Geometry check sheet. Reference: the model listing, model coordinates, mm. A direction names the side the tool comes from. Round coordinates to 2 decimals unless told otherwise and drop trailing zeros. Write each loop counter-clockwise with the first axis right and the second up, starting at its lowest first coordinate (ties: lowest second). Pieces come first, ordered by that corner, then holes. Notation, with made-up numbers: M 18.25,36.5 L 26.25,36.5 A21 ccw 26.25,44.5 Z; hole C -30,51 d8. An arc over 180 degrees is marked long. Use a Markdown table: item, result.
```python
from build123d import *

# Parameters (mm, degrees)
SKETCH1_R           = 6.477
SKETCH1_R_2         = 3.175
BOSS_EXTRUDE1_DEPTH = 228.6
SKETCH2_W           = 12.954
SKETCH2_H           = 7.9375
CUT_EXTRUDE1_DEPTH  = 229.783441398


with BuildPart() as part:
    # Sketch1 → Boss-Extrude1 (new body)
    with BuildSketch(Plane.XY):
        Circle(SKETCH1_R)
        Circle(SKETCH1_R_2, mode=Mode.SUBTRACT)
    extrude(amount=BOSS_EXTRUDE1_DEPTH)

    # Sketch2 → Cut-Extrude1 (cut, through all)
    with BuildSketch(Plane(origin=(0, 0, 0), x_dir=(1, 0, 0), z_dir=(0, 1, 0))):
        with Locations((0, -188.11875)):
            Rectangle(SKETCH2_W, SKETCH2_H)
    extrude(amount=-CUT_EXTRUDE1_DEPTH, mode=Mode.SUBTRACT)


solid = part.part
```
Item 1: Cross-section at B-B, the plane z = 174. Record the cut outline in (x, y) (3 decimals).
Outcome:
| item | result |
|---|---|
| outline | C 0,0 d12.954; hole C 0,0 d6.35 |
Item 2: Access from +Z, -Z, +X, -X, +Y, -Y to the whole of each face (thin tool, end or side, straight path). Record for faces 5 (the face through (-0.843, 6.422, 112.7)), 6 (the face through (0, -4, 184.15)).
Outcome:
| item | result |
|---|---|
| face 5 | +Z, -Z |
| face 6 | +X, -X, -Y |
Item 3: Mould release check, pull along Z, two halves, no side actions. Record for faces 1 (the face through (-0.41, 3.15, 112.7)), 2 (the face through (0, -4, 192.088)), 3 (the face through (3, 2, 0)), 4 (the face through (3, 2, 228.6)): +Z half, -Z half, draft (parallel to the pull), parting line (faces both ways), or undercut.
Outcome:
| item | result |
|---|---|
| face 1 | draft |
| face 2 | undercut |
| face 3 | -Z half |
| face 4 | +Z half |
Item 4: Material ranges on line 1 along Z through (x, y) = (-4.5, -3); line 2 along Y through (x, z) = (0, 170) (3 decimals), recorded low to high. Write a range as from..to.
Outcome:
| item | result |
|---|---|
| line 1 | z = 0..184.15, 192.09..228.6 |
| line 2 | y = -6.477..-3.175, 3.175..6.477 |
Item 5: Cross-section at A-A, the plane x = 0. Count the separate pieces of the cut face and the enclosed holes in it, and give its area (3 significant figures).
Outcome:
| item | result |
|---|---|
| separate pieces | 3 |
| enclosed holes | 0 |
| area | 1,480 mm2 |
Item 6: Go/stop test with flat-tipped pins: pin 1 (2 mm diameter, centred on y = -3, z = 43.5, fed in from +X); pin 2 (3.5 mm diameter, centred on x = 4.5, z = 186.5, fed in from -Y); pin 3 (1 mm diameter, centred on x = -1, z = 204, fed in from +Y). Record where each tip stops, or that it passes through.
Outcome:
| item | result |
|---|---|
| pin 1 | stops at x = 6.16 |
| pin 2 | stops at y = 0 |
| pin 3 | stops at y = 6.46 |
